from build123d import *

# Parameters (mm, degrees)
SCREWHOOK_DEPTH        = 2.54
SPACERANDTOPHOOK_DEPTH = 6.980143326


with BuildPart() as part:
    # Sketch1 → ScrewHook (new body)
    with BuildSketch(Plane(origin=(0, 0, 0), x_dir=(1, 0, 0), z_dir=(0, 1, 0))):
        with BuildLine():
            Line((-5.624189629, 11.672719973), (-19.949200128, 11.672719973))
            Line((-19.949200128, 11.672719973), (-19.949200128, 18.652863299))
            Line((-19.949200128, 18.652863299), (-5.624189629, 18.652863299))
            Line((-5.624189629, 18.652863299), (-5.624189629, 17.065363299))
            ThreePointArc((-5.624189629, 17.065363299), (-5.700318254, 16.884041007), (-5.883069737, 16.811410184))
            Line((-5.883069737, 16.811410184), (-9.311436788, 16.877291636))
            ThreePointArc((-9.311436788, 16.877291636), (-11.059200128, 15.162791636), (-9.311436788, 13.448291636))
            Line((-9.311436788, 13.448291636), (-5.883069737, 13.514173088))
            ThreePointArc((-5.883069737, 13.514173088), (-5.700318254, 13.441542265), (-5.624189629, 13.260219973))
            Line((-5.624189629, 13.260219973), (-5.624189629, 11.672719973))
        make_face()
    extrude(amount=SCREWHOOK_DEPTH)

    # Sketch3 → SpacerAndTopHook (add)
    with BuildSketch(Plane.XY.offset(-11.672719973)):
        Polygon((-19.949200128, 2.54), (-19.949200128, 44.069), (-13.599200128, 44.069), (-13.599200128, 40.894), (-16.774200128, 40.894), (-16.774200128, 27.94), (-13.599200128, 27.94), (-13.599200128, 2.54), align=None)
    extrude(amount=-SPACERANDTOPHOOK_DEPTH)


solid = part.part
The listing builds one solid part. Answer for the finished solid, in the listing's coordinates (mm). A direction names the side the tool comes from. Give positions to 0.01 mm unless a question says otherwise; leave off trailing zeros. Write each loop counter-clockwise with the first axis right and the second up, starting at its lowest first coordinate (ties: lowest second). Pieces come first, ordered by that corner, then holes.
Item 1: Find the intervals of material crossed by line 1 along X through (y, z) = (29.5, -12.5); line 2 along Y through (x, z) = (-12, -12.75); line 3 along X through (y, z) = (20, -16.75), in increasing order.
Item 2: Section B-B, the plane z = -14.75 is taken. Write down the section's boundary in (x, y), plus the area to 3 significant figures.
Item 3: Flat-ended cylindrical pins translate along their axes: P1, Ø2, axis at y = 6, z = -14.5, coming from the +X side; P2, Ø3.5, axis at y = 34.5, z = -15, coming from the +X side. Find the tip coordinate at first contact, or state that the pin passes through.
Item 4: Section D-D, the plane x = -12 is taken. Write down the section's boundary in (y, z).
Item 5: Determine the mould class of faces 1 (the flat face through (-14, 0, -15)), 2 (the flat face through (-19.949, 22, -15)), 3 (the flat face through (-5.624, 1, -12)) for opening direction X: released by +X, released by -X, zero draft, split by the parting line, or undercut.
Item 6: Which of the six approach directions +Z, -Z, +X, -X, +Y, -Y give full straight-line access (tool end or side, diameter ignored) to faces 4 (the flat face through (-15, 40.894, -15)), 5 (the cylindrical face through (-11.06, 1.25, -15.2)), 6 (the flat face through (-13.599, 15, -15))?
Item 7: Section A-A, the plane x = -14.75 is taken. Write down the section's boundary in (y, z), plus the area to 3 significant figures.
Item 8: Section C-C, the plane y = 9.5 is taken. Write down the section's boundary in (x, z).
Completed:
1. line 1: x = -19.95 to -16.77
1. line 2: y = 0 to 2.54
1. line 3: x = -19.95 to -13.6
2. outline: (-19.95, 0) - (-11.01, 0) - (-11.01, 2.54) - (-13.6, 2.54) - (-13.6, 27.94) - (-16.77, 27.94) - (-16.77, 40.89) - (-13.6, 40.89) - (-13.6, 44.07) - (-19.95, 44.07) - close
2. area: 245 mm2
3. P1: stops at x = -13.6
3. P2: stops at x = -16.77
4. outline: (0, -18.65) - (2.54, -18.65) - (2.54, -11.67) - (0, -11.67) - close
5. face 1: zero draft
5. face 2: released by -X
5. face 3: released by +X
6. face 4: +Z, -Z, +X
6. face 5: +Y, -Y
6. face 6: +Z, -Z, +X, +Y
7. outline: (0, -18.65) - (27.94, -18.65) - (27.94, -11.67) - (0, -11.67) - close; (40.89, -18.65) - (44.07, -18.65) - (44.07, -11.67) - (40.89, -11.67) - close
7. area: 217 mm2
8. outline: (-19.95, -18.65) - (-13.6, -18.65) - (-13.6, -11.67) - (-19.95, -11.67) - close
